Check sheet for the modelled part. Datum: model origin and axes. Units: mm. Face numbers are marked on the shaded views. A direction names the side the tool comes from. Round coordinates to 2 decimals unless told otherwise and drop trailing zeros. Write each loop counter-clockwise with the first axis right and the second up, starting at its lowest first coordinate (ties: lowest second). Pieces come first, ordered by that corner, then holes. Notation, with made-up numbers: (10.5, -29.75) - (29.5, -29.75) arc R28 cw to (29.5, 7.25) - close; hole circle Ø7 at (60.25, 86.25). An arc over 180 degrees is marked (long way). Use one line per item in the form item = value. Start each with the question number.
1) Section check C-C (z = 16.5). Count the separate pieces of the cut face and the enclosed holes in it, then the cut area to 3 significant figures.
2) Set-up check for the marked faces 1 and 2: record each of +Z, -Z, +X, -X, +Y, -Y from which the full face is reachable in a straight line by a thin tool's end or side.
3) Section check A-A (x = -12.5). Record the boundary of the cut face in (y, z), then the cut area to 3 significant figures.
4) Gauge pin test, flat ends, axial feed: P1, Ø14.5, axis at x = -34.5, z = 10, coming from the +Y side; P2, Ø12, axis at y = 28.5, z = 19, coming from the -X side; P3, Ø8, axis at x = -26, y = 16, coming from the +Z side. Record the tip position at first contact, or that the pin passes through.
5) Section check D-D (x = -1.5). Record the boundary of the cut face in (y, z).
6) Scan lines: probe 1 along Z at (x, y) = (2.05, 30); probe 2 along X at (y, z) = (-13.5, 3); probe 3 along Z at (x, y) = (2, -7). Record each from-to range of solid material in increasing order.
7) Section check B-B (y = -7.5). Record the boundary of the cut face in (x, z).
from build123d import *

# Parameters (mm, degrees)
F0_W          = 50
F0_H          = 4
F0_R          = 1.5
F1_DEPTH      = 3
F2_DEPTH      = 50
F2_DEPTH_BACK = 3
F0_W_2        = 40
F3_DEPTH      = 25
F3_DEPTH_BACK = 3
F4_R          = 1.5
F5_DEPTH      = 25


with BuildPart() as f1:
    # F0 (on Right) → F1 (new body)
    with BuildSketch(Plane.YZ):
        with Locations((-20, 2)):
            Rectangle(F0_W, F0_H)
        Polygon((-45, 29), (-45, 4), (5, 4), (45, 4), (45, 29), align=None)
        with Locations((-32.5, 16.5)):
            Circle(F0_R, mode=Mode.SUBTRACT)
        with Locations((-7.5, 16.5)):
            Circle(F0_R, mode=Mode.SUBTRACT)
        with Locations((17.5, 16.5)):
            Circle(F0_R, mode=Mode.SUBTRACT)
        with Locations((30, 16.5)):
            Circle(F0_R, mode=Mode.SUBTRACT)
        with Locations((42.5, 16.5)):
            Circle(F0_R, mode=Mode.SUBTRACT)
    extrude(amount=F1_DEPTH)

    # F0 (on Right) → F2 (join, two sides)
    with BuildSketch(Plane.YZ) as f2_sk:
        Polygon((-45, 0), (-45, 4), (-45, 29), (-50.000000447, 29), (-50.000000447, 0), align=None)
    extrude(amount=-F2_DEPTH)
    extrude(f2_sk.sketch, amount=F2_DEPTH_BACK)

    # F0 (on Right) → F3 (join, two sides)
    with BuildSketch(Plane.YZ) as f3_sk:
        with Locations((25, 2)):
            Rectangle(F0_W_2, F0_H)
    extrude(amount=-F3_DEPTH)
    extrude(f3_sk.sketch, amount=F3_DEPTH_BACK)

    # F4 (on face) → F5 (cut)
    with BuildSketch(Plane.XZ.offset(50.000000447)):
        with Locations((-37.5, 16.5)):
            Circle(F4_R)
        with Locations((-12.5, 16.5)):
            Circle(F4_R)
    extrude(amount=-F5_DEPTH, mode=Mode.SUBTRACT)


solid = f1.part
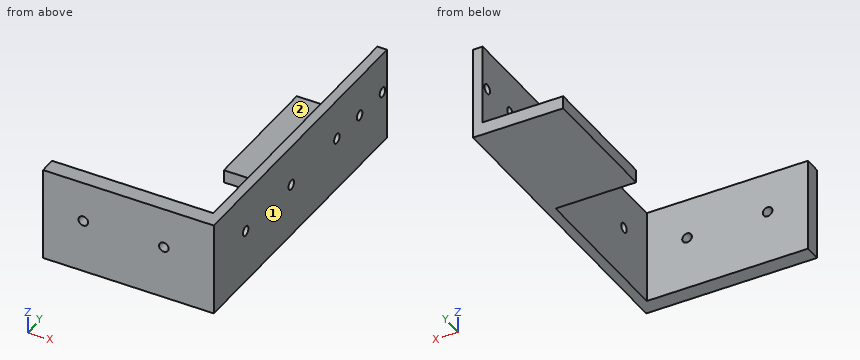
Results are:
q1.separate_pieces = 8
q1.enclosed_holes = 0
q1.area = 460 mm²
q2.face_1 = +Z, -Z, +X, +Y, -Y
q2.face_2 = +Z, -X, +Y
q3.outline = (-50, 0) - (-45, 0) - (-45, 15) - (-50, 15) - close; (-50, 18) - (-45, 18) - (-45, 29) - (-50, 29) - close; (5, 0) - (45, 0) - (45, 4) - (5, 4) - close
q3.area = 290 mm²
q4.P1 = -45
q4.P2 = 0
q4.P3 = 4
q5.outline = (-50, 0) - (-45, 0) - (-45, 29) - (-50, 29) - close; (5, 0) - (45, 0) - (45, 4) - (5, 4) - close
q6.probe_1 = 0 to 15, 18 to 29
q6.probe_2 = 0 to 3
q6.probe_3 = 0 to 15.09, 17.91 to 29
q7.outline = (0, 0) - (3, 0) - (3, 15) - (0, 15) - close; (0, 18) - (3, 18) - (3, 29) - (0, 29) - close
